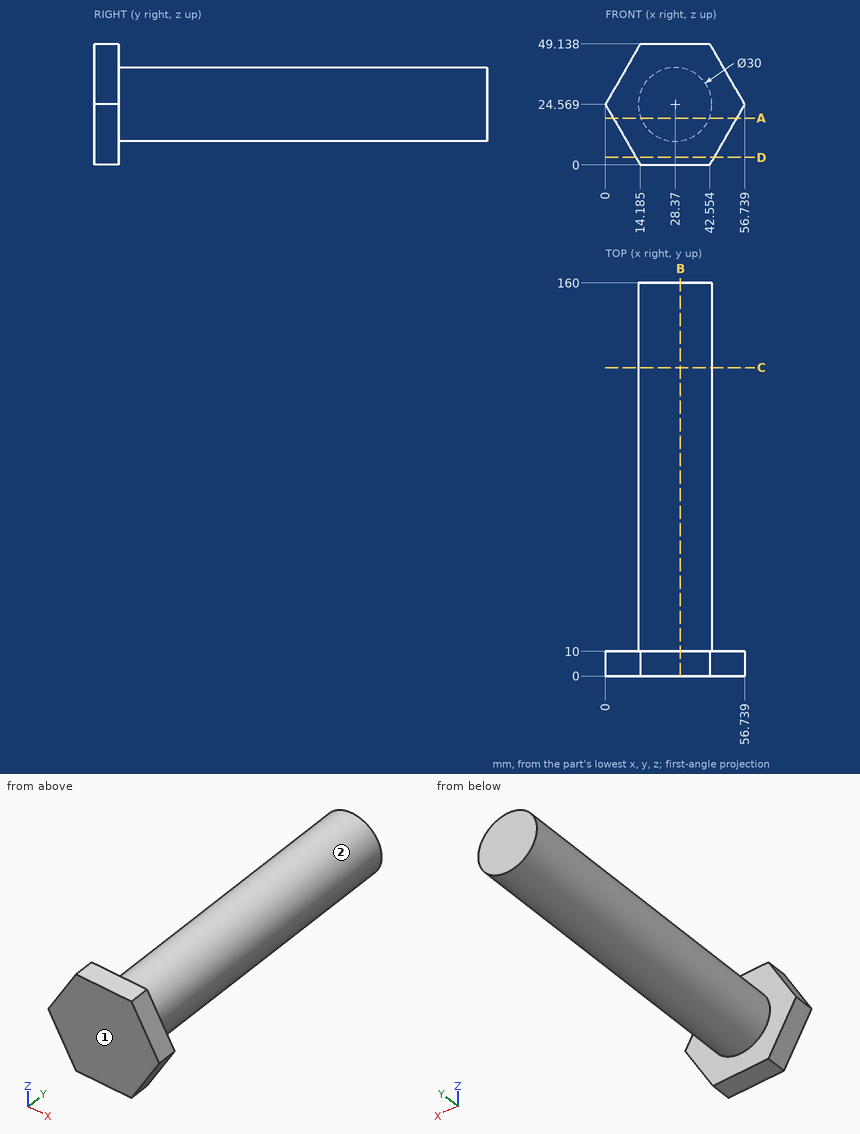
Input: dimensioned drawing with shaded views. Units: mm. Origin: part minimum x, y, z. A direction names the side the tool comes from. Give positions to 0.01 mm unless a question says otherwise; leave off trailing zeros. Order: outer loops, then holes, each group sorted by start corner. A loop starts at its lowest first (then second) coordinate and runs counter-clockwise, first axis right, second up.
(1) Access query for the marked faces 1 and 2. Directions: +Z, -Z, +X, -X, +Y, -Y. A direction counts if a zero-diameter tool reaches every point of the face in a straight line with its end or side. Return the directions, or none.
(2) Material intervals for line 1 along Y through (x, z) = (19.5, 5); line 2 along X through (y, z) = (66, 24); line 3 along Z through (x, y) = (31.5, 87), sorted ascending.
(3) Contact query for flat-ended pins moving along their axis: P1, Ø2, axis at y = 17.5, z = 37.5, coming from the +X side; P2, Ø5, axis at y = 18.5, z = 25.5, coming from the +X side; P3, Ø5, axis at x = 22.5, z = 30, coming from the -Y side; P4, Ø10, axis at y = 93.5, z = 31, coming from the -X side. Output: stop coordinate, or through.
(4) Section query D-D (z = 3). Return the cut outline in (x, y), plus the area to 3 significant figures.
(5) Section query C-C (y = 125.5). Return the cut outline in (x, z), plus the area to 3 significant figures.
(6) Section query A-A (z = 19). Return the cut outline in (x, y) (1 decimal), plus the area to 3 significant figures.
(7) Section query B-B (x = 30.5). Return the cut outline in (y, z), plus the area to 3 significant figures.
Outcome:
1. face 1: +Z, -Z, +X, -X, -Y
1. face 2: +Y
2. line 1: y = 0 to 10
2. line 2: x = 13.38 to 43.36
2. line 3: z = 9.9 to 39.24
3. P1: stops at x = 37.46
3. P2: stops at x = 43.37
3. P3: stops at y = 0
3. P4: stops at x = 13.44
4. outline: (12.45, 0) - (44.29, 0) - (44.29, 10) - (12.45, 10) - close
4. area: 318 mm2
5. outline: circle Ø30 at (28.37, 24.57)
5. area: 707 mm2
6. outline: (3.2, 0) - (53.5, 0) - (53.5, 10) - (42.3, 10) - (42.3, 160) - (14.4, 160) - (14.4, 10) - (3.2, 10) - close
6. area: 4,680 mm2
7. outline: (0, 0) - (10, 0) - (10, 9.72) - (160, 9.72) - (160, 39.42) - (10, 39.42) - (10, 49.14) - (0, 49.14) - close
7. area: 4,950 mm2
